Can you work these out from the model? Positions are in its coordinate system, mm. Give positions to 0.01 mm unless a question says otherwise; leave off trailing zeros. Loops run counter-clockwise (first coordinate to the right, second up) from the corner with the lowest first, then second, coordinate; pieces in that order, holes last. Notation, with made-up numbers: (21, -4) -> (33, -4) arc R28 ccw to (33, 15) -> close; hole circle Ø2 at (-6, 88.25). An arc over 180 degrees is marked (long way). One line per question, with ' | ' between items.
from build123d import *

# Parameters (mm, degrees)
FILLET1_R          = 2.159
SKETCH3_R          = 2.413
CUT_EXTRUDE1_DEPTH = 21.59


with BuildPart() as part:
    # Sketch1 → Revolve1 (revolve)
    with BuildSketch(Plane.XY, mode=Mode.PRIVATE) as revolve1_sk:
        Polygon((0, 0), (0, 2.8), (1.48625, 4.28625), (21.59, 4.28625), (21.59, 0), align=None)
    revolve(revolve1_sk.sketch.rotate(Axis((0, 0, 0), (1, 0, 0)), 90), axis=Axis((0, 0, 0), (1, 0, 0)))

    # Fillet1
    fillet1_edges = [part.edges().sort_by_distance(p)[0] for p in [
        (1.48625, 0, -4.28625),
    ]]
    fillet(fillet1_edges, radius=FILLET1_R)

    # Sketch3 → Cut-Extrude1 (cut)
    with BuildSketch(Plane.ZY):
        Circle(SKETCH3_R)
    extrude(amount=-CUT_EXTRUDE1_DEPTH, mode=Mode.SUBTRACT)


solid = part.part
Q1. If we mould it in two halves opening along Y, with no side actions, what happens to faces 1 (the face through (10.644, -1.468, -1.915)), 2 (the face through (12.12, 1.64, 3.96)), 3 (the face through (21.59, 2, 2))? For each: pulls with the +Y half, pulls with the -Y half, needs draft (parallel to the pull), parting line crosses it, or undercut.
Entries:
face 1: undercut | face 2: parting line crosses it | face 3: needs draft
Q2. If I drill on probe 1 along Y at (x, z) = (14.75, 0); probe 2 along Z at (x, y) = (1.25, -1.75); probe 3 along Z at (x, y) = (14.5, 1), over which ranges is the centre line in solid material (lowest first)? Write a range as from..to.
Entries:
probe 1: -4.29..-2.41, 2.41..4.29 | probe 2: -3.56..-1.66, 1.66..3.56 | probe 3: -4.17..-2.2, 2.2..4.17
Q3. If we section it at A-A (x = 10.25): Write out the boundary of the cut face in (y, z), plus the area to 3 significant figures.
Entries:
outline: circle Ø8.57 at (0, 0); hole circle Ø4.83 at (0, 0) | area: 39.4 mm²
Q4. For pin 1 Ø1.5 at (x, y) = (16, 2.5) entering from +Z, with a flat end and sliding along its axis, tell me the tip position at first contact or that it passes through.
Entries:
pin 1: z = 3.91
